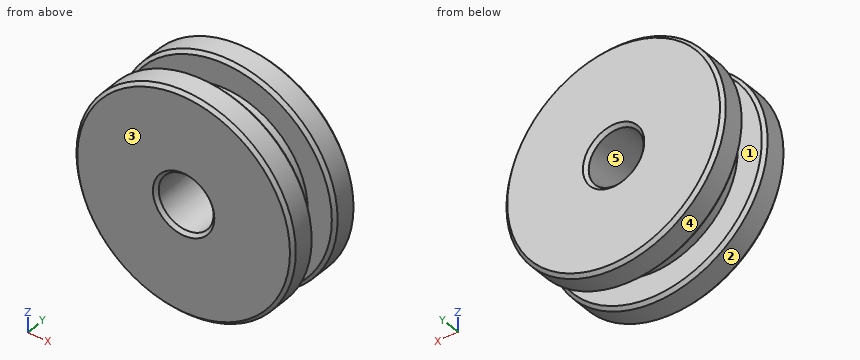
from build123d import *

# Parameters (mm, degrees)
F2_R     = 3.175
F3_DEPTH = 9.526
F4_SIZE  = 0.381


with BuildPart() as f1:
    # F0 (on Top) → F1 (revolve)
    with BuildSketch(Plane.XY):
        Polygon((0, 9.525), (0, 0), (12.7, 0), (12.7, 3.175), (9.525, 3.175), (9.525, 6.35), (12.7, 6.35), (12.7, 9.525), align=None)
    revolve(axis=Axis((0, 4.7625, 0), (0, 1, 0)))

    # F2 (on face) → F3 (cut, through all)
    with BuildSketch(Plane.XZ):
        Circle(F2_R)
    extrude(amount=-F3_DEPTH, mode=Mode.SUBTRACT)

    # F4
    f4_edges = [f1.edges().sort_by_distance(p)[0] for p in [
        (-3.175, 0, 0),
        (-3.175, 9.525, 0),
        (-12.7, 0, 0),
        (-12.7, 3.175, 0),
        (-12.7, 6.35, 0),
        (-12.7, 9.525, 0),
    ]]
    chamfer(f4_edges, length=F4_SIZE)


solid = f1.part
For this review, take the finished solid that the model builds, in its own axes (mm). Face numbers are marked on the shaded views. A direction names the side the tool comes from. Round coordinates to 2 decimals unless told otherwise and drop trailing zeros. Loops run counter-clockwise (first coordinate to the right, second up) from the corner with the lowest first, then second, coordinate; pieces in that order, holes last. Notation, with made-up numbers: (-5, 72) - (5, 72) arc R9 ccw to (5, 77) - close; hole circle Ø6 at (77.5, 63). An arc over 180 degrees is marked (long way). Put each result on its own line as item: value. Start each with the question number.
1. Consider section C-C on y = 4.75. State the section outline as (x, z) points (3 decimals).
2. Mouldability with a two-part tool opening along X and no side actions: class the marked faces 3, 4 and 5 as +X half, -X half, draft (parallel to the pull), parting line (faces both ways), or undercut.
3. For probe 1 along Y at (x, z) = (-11, 2.5) (3 decimals); probe 2 along Z at (x, y) = (0, 6.25) (3 decimals); probe 3 along Z at (x, y) = (0, 7) (3 decimals), list the stretches that pass through material, from the lowest coordinate up. Write a range as [from, to].
4. Insertion check: P1, Ø1.5, axis at y = 3, z = 2.5, coming from the +X side; P2, Ø1, axis at x = 5.5, y = 4, coming from the -Z side; P3, Ø1.5, axis at x = 0.5, z = -7, coming from the -Y side; P4, Ø3, axis at x = -8.5, y = 2.5, coming from the +Z side. Each pin has a flat end and moves straight along its axis. Give the tip position at first contact, or say it passes through.
5. Consider section B-B on x = 0. State the section outline as (y, z) points (3 decimals).
6. For the marked faces 1 and 2, list the 3-axis set-ups (+Z, -Z, +X, -X, +Y, -Y) from which the entire face can be reached by the end or side of a thin tool; tool diameter is ignored.
7. Consider section A-A on z = 0. State the section outline as (x, y) points (3 decimals).
8. Consider section D-D on y = 2.25. State the section outline as (x, z) points (3 decimals), plus the area to 3 significant figures.
Result sheet:
1. outline: circle Ø19.05 at (0, 0); hole circle Ø6.35 at (0, 0)
2. face 3: draft
2. face 4: parting line
2. face 5: undercut
3. probe 1: [0, 3.175], [6.35, 9.525]
3. probe 2: [-9.525, -3.175], [3.175, 9.525]
3. probe 3: [-12.7, -3.175], [3.175, 12.7]
4. P1: x = 12.57
4. P2: z = -8.11
4. P3: y = 0
4. P4: z = 10.6
5. outline: (0, -12.319) - (0.381, -12.7) - (2.794, -12.7) - (3.175, -12.319) - (3.175, -9.525) - (6.35, -9.525) - (6.35, -12.319) - (6.731, -12.7) - (9.144, -12.7) - (9.525, -12.319) - (9.525, -3.556) - (9.144, -3.175) - (0.381, -3.175) - (0, -3.556) - close; (0, 3.556) - (0.381, 3.175) - (9.144, 3.175) - (9.525, 3.556) - (9.525, 12.319) - (9.144, 12.7) - (6.731, 12.7) - (6.35, 12.319) - (6.35, 9.525) - (3.175, 9.525) - (3.175, 12.319) - (2.794, 12.7) - (0.381, 12.7) - (0, 12.319) - close
6. face 1: none
6. face 2: +Y, -Y
7. outline: (-12.7, 0.381) - (-12.319, 0) - (-3.556, 0) - (-3.175, 0.381) - (-3.175, 9.144) - (-3.556, 9.525) - (-12.319, 9.525) - (-12.7, 9.144) - (-12.7, 6.731) - (-12.319, 6.35) - (-9.525, 6.35) - (-9.525, 3.175) - (-12.319, 3.175) - (-12.7, 2.794) - close; (3.175, 0.381) - (3.556, 0) - (12.319, 0) - (12.7, 0.381) - (12.7, 2.794) - (12.319, 3.175) - (9.525, 3.175) - (9.525, 6.35) - (12.319, 6.35) - (12.7, 6.731) - (12.7, 9.144) - (12.319, 9.525) - (3.556, 9.525) - (3.175, 9.144) - close
8. outline: circle Ø25.4 at (0, 0); hole circle Ø6.35 at (0, 0)
8. area: 475 mm^2
